from build123d import *

# Parameters (mm, degrees)
SKETCH1_W            = 78.74
SKETCH1_H            = 66.04
SKETCH1_W_2          = 71.12
SKETCH1_H_2          = 55.88
BOSS_EXTRUDE1_DEPTH  = 63.5
SKETCH2_W            = 78.74
SKETCH2_H            = 66.04
BOSS_EXTRUDE2_DEPTH  = 4
CUT_EXTRUDE1_REACH   = 120.103
SKETCH3_W            = 13.462
SKETCH3_H            = 13.97
CUT_EXTRUDE2_REACH   = 120.103
SKETCH4_W            = 10.922
SKETCH4_H            = 13.97
SKETCH16_W           = 66.04
SKETCH16_H           = 67.5
SKETCH16_W_2         = 13.462
SKETCH16_H_2         = 13.97
SKETCH16_W_3         = 10.922
BOSS_EXTRUDE8_DEPTH  = 3
SKETCH17_W           = 81.74
SKETCH17_H           = 66.04
BOSS_EXTRUDE9_DEPTH  = 4
CUT_EXTRUDE10_DEPTH  = 64.77
SKETCH19_W           = 2.5
SKETCH19_H           = 60.96
CUT_EXTRUDE11_DEPTH  = 3
SKETCH20_W           = 55.88
SKETCH20_H           = 4
BOSS_EXTRUDE10_DEPTH = 2.25
SKETCH21_W           = 71.12
SKETCH21_H           = 55.88
BOSS_EXTRUDE11_DEPTH = 2.73
FILLET2_R            = 0.5
BOSS_EXTRUDE12_DEPTH = 6.35
SKETCH22_R           = 10.16
CUT_EXTRUDE12_DEPTH  = 11.35
CUT_EXTRUDE13_DEPTH  = 2
FILLET3_R            = 2.5


with BuildPart() as part:
    # Sketch1 → Boss-Extrude1 (new body)
    with BuildSketch(Plane(origin=(0, 0, 0), x_dir=(1, 0, 0), z_dir=(0, 1, 0))):
        with Locations((35.56, 27.94)):
            Rectangle(SKETCH1_W, SKETCH1_H)
        with Locations((35.56, 27.94)):
            Rectangle(SKETCH1_W_2, SKETCH1_H_2, mode=Mode.SUBTRACT)
    extrude(amount=BOSS_EXTRUDE1_DEPTH)

    # Sketch2 → Boss-Extrude2 (add)
    with BuildSketch(Plane(origin=(0, 0, 0), x_dir=(1, 0, 0), z_dir=(0, 1, 0))):
        with Locations((35.56, 27.94)):
            Rectangle(SKETCH2_W, SKETCH2_H)
    extrude(amount=-BOSS_EXTRUDE2_DEPTH)

    # Sketch3 → Cut-Extrude1 (cut, up to next)
    with BuildSketch(Plane.ZY.offset(3.81), mode=Mode.PRIVATE) as cut_extrude1_sk1:
        with Locations((-40.729, 11.875)):
            Rectangle(SKETCH3_W, SKETCH3_H)
    cut_extrude1_tool1 = extrude(cut_extrude1_sk1.sketch, amount=-CUT_EXTRUDE1_REACH, mode=Mode.PRIVATE) & part.part
    add(cut_extrude1_tool1.solids().sort_by_distance((-3.81, 11.875, -40.729))[0], mode=Mode.SUBTRACT)

    # Sketch4 → Cut-Extrude2 (cut, up to next)
    with BuildSketch(Plane.ZY.offset(3.81), mode=Mode.PRIVATE) as cut_extrude2_sk1:
        with Locations((-8.001, 11.875)):
            Rectangle(SKETCH4_W, SKETCH4_H)
    cut_extrude2_tool1 = extrude(cut_extrude2_sk1.sketch, amount=-CUT_EXTRUDE2_REACH, mode=Mode.PRIVATE) & part.part
    add(cut_extrude2_tool1.solids().sort_by_distance((-3.81, 11.875, -8.001))[0], mode=Mode.SUBTRACT)

    # Sketch16 → Boss-Extrude8 (add)
    with BuildSketch(Plane.ZY.offset(3.81)):
        with Locations((-27.94, 29.75)):
            Rectangle(SKETCH16_W, SKETCH16_H)
        with Locations((-40.729, 11.875)):
            Rectangle(SKETCH16_W_2, SKETCH16_H_2, mode=Mode.SUBTRACT)
        with Locations((-8.001, 11.875)):
            Rectangle(SKETCH16_W_3, SKETCH16_H_2, mode=Mode.SUBTRACT)
    extrude(amount=BOSS_EXTRUDE8_DEPTH)

    # Sketch17 → Boss-Extrude9 (add)
    with BuildSketch(Plane(origin=(0, 63.5, 0), x_dir=(1, 0, 0), z_dir=(0, 1, 0))):
        with Locations((34.06, 27.94)):
            Rectangle(SKETCH17_W, SKETCH17_H)
    extrude(amount=BOSS_EXTRUDE9_DEPTH)

    # Sketch18 → Cut-Extrude10 (cut)
    with BuildSketch(Plane(origin=(0, 67.5, 0), x_dir=(1, 0, 0), z_dir=(0, 1, 0))):
        Polygon((-4.560006, 58.42), (-2.060006, 58.42), (-2.060006, 55.88), (0.189988, 55.88), (0.189988, 0), (-2.060006, 0), (-2.060006, -2.54), (-4.560006, -2.54), (-4.560006, 0), (-6.81, 0), (-6.81, 55.88), (-4.560006, 55.88), align=None)
    extrude(amount=-CUT_EXTRUDE10_DEPTH, mode=Mode.SUBTRACT)

    # Sketch19 → Cut-Extrude11 (cut)
    with BuildSketch(Plane(origin=(0, 2.73, 0), x_dir=(1, 0, 0), z_dir=(0, 1, 0))):
        with Locations((-3.310006, 27.94)):
            Rectangle(SKETCH19_W, SKETCH19_H)
    extrude(amount=-CUT_EXTRUDE11_DEPTH, mode=Mode.SUBTRACT)

    # Sketch20 → Boss-Extrude10 (add)
    with BuildSketch(Plane.ZY.offset(-0.189988)):
        with Locations((-27.94, 65.5)):
            Rectangle(SKETCH20_W, SKETCH20_H)
    extrude(amount=BOSS_EXTRUDE10_DEPTH)

    # Sketch21 → Boss-Extrude11 (add)
    with BuildSketch(Plane(origin=(0, 0, 0), x_dir=(1, 0, 0), z_dir=(0, 1, 0))):
        with Locations((35.56, 27.94)):
            Rectangle(SKETCH21_W, SKETCH21_H)
    extrude(amount=BOSS_EXTRUDE11_DEPTH)

    # Fillet2
    fillet2_edges = [part.edges().sort_by_distance(p)[0] for p in [
        (-2.060006, 33.615, -58.42),
    ]]
    fillet(fillet2_edges, radius=FILLET2_R)
    fillet2_2_edges = [part.edges().sort_by_distance(p)[0] for p in [
        (-2.060006, -0.27, -27.69),
    ]]
    fillet(fillet2_2_edges, radius=FILLET2_R)
    fillet2_3_edges = [part.edges().sort_by_distance(p)[0] for p in [
        (-2.060006, 33.865, 2.54),
    ]]
    fillet(fillet2_3_edges, radius=FILLET2_R)
    fillet2_4_edges = [part.edges().sort_by_distance(p)[0] for p in [
        (-4.560006, 33.865, 2.54),
    ]]
    fillet(fillet2_4_edges, radius=FILLET2_R)
    fillet2_5_edges = [part.edges().sort_by_distance(p)[0] for p in [
        (-3.310006, 67.5, 2.54),
    ]]
    fillet(fillet2_5_edges, radius=FILLET2_R)
    fillet2_6_edges = [part.edges().sort_by_distance(p)[0] for p in [
        (-4.560006, 67.5, -56.9),
    ]]
    fillet(fillet2_6_edges, radius=FILLET2_R)
    fillet2_7_edges = [part.edges().sort_by_distance(p)[0] for p in [
        (-2.060012, 67.5, -27.94),
    ]]
    fillet(fillet2_7_edges, radius=FILLET2_R - 0.0001)  # a hair under: the kernel refuses the full size

    # Sketch11 → Boss-Extrude12 (add)
    with BuildSketch(Plane.XY.offset(5.08)):
        Polygon((49.81, 46.327241336), (49.81, 29.872758664), (35.56, 21.645517328), (21.31, 29.872758664), (21.31, 46.327241336), (35.56, 54.554482672), align=None)
    extrude(amount=BOSS_EXTRUDE12_DEPTH)

    # Sketch22 → Cut-Extrude12 (cut)
    with BuildSketch(Plane.XY.offset(11.43)):
        with Locations((35.56, 38.1)):
            Circle(SKETCH22_R)
    extrude(amount=-CUT_EXTRUDE12_DEPTH, mode=Mode.SUBTRACT)

    # Sketch23 → Cut-Extrude13 (cut)
    with BuildSketch(Plane(origin=(0, 0, 0), x_dir=(-1, 0, 0), z_dir=(0, 0, -1))):
        Polygon((-21.31, 46.327241336), (-21.31, 29.872758664), (-35.56, 21.645517328), (-49.81, 29.872758664), (-49.81, 46.327241336), (-35.56, 54.554482672), align=None)
    extrude(amount=-CUT_EXTRUDE13_DEPTH, mode=Mode.SUBTRACT)

    # Fillet3
    fillet3_edges = [part.edges().sort_by_distance(p)[0] for p in [
        (42.685, 50.440862004, 5.08),
        (28.435, 50.440862004, 5.08),
        (21.31, 38.1, 5.08),
        (28.435, 25.759137996, 5.08),
        (42.685, 25.759137996, 5.08),
        (49.81, 38.1, 5.08),
    ]]
    fillet(fillet3_edges, radius=FILLET3_R)


solid = part.part
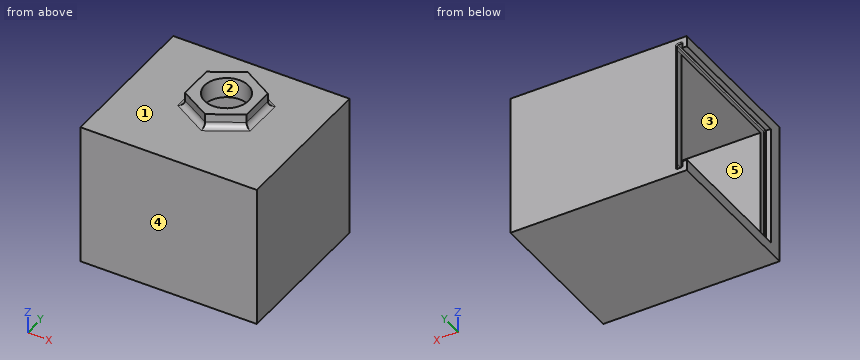
Could you check a few things on this model? Use its own coordinates, in mm. Face numbers are marked on the shaded views. A direction names the side the tool comes from. Coordinates: 2 decimals unless noted, no trailing zeros. Order: outer loops, then holes, each group sorted by start corner. A loop starts at its lowest first (then second) coordinate and runs counter-clockwise, first axis right, second up. Notation, with made-up numbers: (80.5, 25) -> (120.5, 25) arc R16 ccw to (120.5, 47) -> close; hole circle Ø5 at (75, 13). An arc over 180 degrees is marked (long way). One line per item, written item: value. Start each with the question number.
1) Imagine slicing it at B-B on x = 3.5. List the corners of the cut face in (y, z) for me.
2) If I drill on L1, parallel to X at y = 41, z = 1; L2, parallel to Y at x = 62.5, z = -50; L3, parallel to Z at x = 67, y = 57, over which ranges is the centre line in solid material (lowest first)? Write a range as [from, to].
3) I'm going to push flat-ended pins straight in: pin 1 (2.5 mm diameter, centred on x = -5.5, y = 51, fed in from +Z); pin 2 (2 mm diameter, centred on y = 28.5, z = -43.5, fed in from -X); pin 3 (2.5 mm diameter, centred on x = -5.5, z = -20.5, fed in from +Y). Where does each tip first touch, or does it pass through?
4) Which directions (+Z, -Z, +X, -X, +Y, -Y) give clear straight access to the entire face, cutting with the end or side of a thin tool? Please do the marked faces 4 and 5.
5) We'd pull the mould along Z, two halves only. Please class the marked faces 1, 2 and 3: +Z half, -Z half, draft (parallel to the pull), parting line (faces both ways), or undercut.
6) Imagine slicing it at C-C on z = -32.5. List the corners of the cut face in (x, y) for me.
7) Imagine slicing it at D-D on y = 4. List the corners of the cut face in (x, z) for me.
Answer list:
1. outline: (-4, -60.96) -> (67.5, -60.96) -> (67.5, 5.08) -> (-4, 5.08) -> close; hole (2.73, -55.88) -> (63.5, -55.88) -> (63.5, 0) -> (2.73, 0) -> close
2. L1: x = [-6.81, -4.56], [-2.06, 21.31], [49.81, 74.93]
2. L2: y = [-4, 2.73], [63.5, 67.5]
2. L3: z = [-60.96, -55.88], [0, 5.08]
3. pin 1: stops at z = 5.08
3. pin 2: stops at x = 71.12
3. pin 3: stops at y = 2.73
4. face 4: +Z, -Z, +X, -X, -Y
4. face 5: -X
5. face 1: +Z half
5. face 2: draft
5. face 3: undercut
6. outline: (-6.81, -4) -> (74.93, -4) -> (74.93, 67.5) -> (-1.56, 67.5) arc R0.5 ccw to (-2.06, 67) -> (-2.06, 63.5) -> (71.12, 63.5) -> (71.12, 2.73) -> (-2.06, 2.73) -> (-2.06, 0.23) arc R0.5 cw to (-2.56, -0.27) -> (-4.06, -0.27) arc R0.5 cw to (-4.56, 0.23) -> (-4.56, 2.73) -> (-6.81, 2.73) -> close
7. outline: (-6.81, -60.96) -> (74.93, -60.96) -> (74.93, 5.08) -> (-6.81, 5.08) -> (-6.81, 0) -> (-4.56, 0) -> (-4.56, 2.04) arc R0.5 cw to (-4.06, 2.54) -> (-2.56, 2.54) arc R0.5 cw to (-2.06, 2.04) -> (-2.06, 0) -> (71.12, 0) -> (71.12, -55.88) -> (-2.06, -55.88) -> (-2.06, -57.92) arc R0.5 cw to (-2.56, -58.42) -> (-4.06, -58.42) arc R0.5 cw to (-4.56, -57.92) -> (-4.56, -55.88) -> (-6.81, -55.88) -> close
